from build123d import *

# Parameters (mm, degrees)
SKETCH_1_W          = 70
SKETCH_1_H          = 12
SKETCH_1_R          = 40
SKETCH_1_R_2        = 35
SKETCH_1_W_2        = 35
EXTRUDE_1_DEPTH     = 12
FILLET_1_R          = 10
SKETCH_2_R          = 2
CUT_EXTRUDE_1_DEPTH = 27
CUT_EXTRUDE_START   = -6
SKETCH_2_3_R        = 4
SKETCH_2_3_R_2      = 2
CUT_EXTRUDE_2_DEPTH = 18
EXTRUDE_START       = -12
EXTRUDE_2_DEPTH     = 12
CUT_EXTRUDE_START_2 = -12
CUT_EXTRUDE_3_DEPTH = 12
SKETCH_4_R          = 2
CUT_EXTRUDE_4_DEPTH = 67.19801074


with BuildPart() as part:
    # 스케치1 → 보스-돌출1 (new body)
    # profile 1 of 7: a face of its own
    with BuildSketch(Plane(origin=(0, 0, 0), x_dir=(0, 0, -1), z_dir=(1, 0, 0))):
        with Locations((0, -46)):
            Rectangle(SKETCH_1_W, SKETCH_1_H)
    # profile 2 of 7: a face of its own
    with BuildSketch(Plane(origin=(0, 0, 0), x_dir=(0, 0, -1), z_dir=(1, 0, 0))):
        Circle(SKETCH_1_R)
        Circle(SKETCH_1_R_2, mode=Mode.SUBTRACT)
    # profile 3 of 7: a face of its own
    with BuildSketch(Plane(origin=(0, 0, 0), x_dir=(0, 0, -1), z_dir=(1, 0, 0))):
        with BuildLine():
            ThreePointArc((-18.119935206, -35.660453561), (-26.285525679, -38.897757113), (-35, -40))
            Line((-35, -40), (0, -40))
            ThreePointArc((0, -40), (-9.316164919, -38.899988062), (-18.119935206, -35.660453561))
        make_face()
    # profile 4 of 7: a face of its own
    with BuildSketch(Plane(origin=(0, 0, 0), x_dir=(0, 0, -1), z_dir=(1, 0, 0))):
        with Locations((17.5, -46)):
            Rectangle(SKETCH_1_W_2, SKETCH_1_H)
    # profile 5 of 7: a face of its own
    with BuildSketch(Plane(origin=(0, 0, 0), x_dir=(0, 0, -1), z_dir=(1, 0, 0))):
        with BuildLine():
            ThreePointArc((18.119935206, -35.660453561), (9.316164919, -38.899988062), (0, -40))
            Line((0, -40), (35, -40))
            ThreePointArc((35, -40), (26.285525679, -38.897757113), (18.119935206, -35.660453561))
        make_face()
    # profile 6 of 7: a face of its own
    with BuildSketch(Plane(origin=(0, 0, 0), x_dir=(0, 0, -1), z_dir=(1, 0, 0))):
        with BuildLine():
            ThreePointArc((-18.119935206, -35.660453561), (-9.316164919, -38.899988062), (0, -40))
            Line((0, -40), (0, -35))
            ThreePointArc((0, -35), (-35, 0), (0, 35))
            Line((0, 35), (0, 40))
            ThreePointArc((0, 40), (-38.899988062, 9.316164919), (-18.119935206, -35.660453561))
        make_face()
    # profile 7 of 7: a face of its own
    with BuildSketch(Plane(origin=(0, 0, 0), x_dir=(0, 0, -1), z_dir=(1, 0, 0))):
        with BuildLine():
            Line((0, -35), (0, -40))
            ThreePointArc((0, -40), (9.316164919, -38.899988062), (18.119935206, -35.660453561))
            ThreePointArc((18.119935206, -35.660453561), (34.093968735, -20.918921958), (40, 0))
            ThreePointArc((40, 0), (28.284271247, 28.284271247), (0, 40))
            Line((0, 40), (0, 35))
            ThreePointArc((0, 35), (24.748737342, 24.748737342), (35, 0))
            ThreePointArc((35, 0), (24.748737342, -24.748737342), (0, -35))
        make_face()
    extrude(amount=EXTRUDE_1_DEPTH)

    # 필렛1
    # the kernel refuses this fillet: 10 mm, written as the material it adds along each edge
    with BuildSketch(Plane(origin=(0, -35.660453561, -18.119935206), x_dir=(0, -0.24898498059862248, -0.9685073460931021), z_dir=(1, 0, 0))) as fillet_1_piece_1:
        with BuildLine():
            CenterArc((19.307998012, 9.821872198), FILLET_1_R, 156.16657794, 103.002878163)
            Line((10.16075687, 13.862661663), (9.977812048, 13.943477452))
            ThreePointArc((9.977812048, 13.943477452), (5.672446884, 6.497369179), (-0.132141038, 0.150129098))
            Line((-0.132141038, 0.150129098), (-0.049796996, -0.193701469))
            ThreePointArc((-0.049796996, -0.193701469), (8.714474321, -1.302242887), (17.391367655, -0.196437444))
            Line((17.391367655, -0.196437444), (17.428948642, 0))
        make_face()
    extrude(amount=12)
    with BuildSketch(Plane(origin=(0, -35.660453561, 18.119935206), x_dir=(0, 0.6339570106071373, 0.7733682878823399), z_dir=(1, 0, 0))) as fillet_1_piece_2:
        with BuildLine():
            CenterArc((19.336075357, 9.766480968), FILLET_1_R, 154.590671351, 103.002878163)
            Line((10.303420921, 14.057303016), (10.122767833, 14.143119457))
            ThreePointArc((10.122767833, 14.143119457), (4.101387619, 7.798494651), (-0.185668093, 0.074346212))
            Line((-0.185668093, 0.074346212), (0.042969056, -0.195329619))
            ThreePointArc((0.042969056, -0.195329619), (8.59381127, 0.734076129), (17.144653483, -0.195329619))
            Line((17.144653483, -0.195329619), (17.187622539, 0))
        make_face()
    extrude(amount=12)

    # 스케치2 → 컷-돌출1 (cut)
    with BuildSketch(Plane.XZ.offset(52)):
        with Locations(Location((6, 0, 0), (0, 0, 270))):
            Circle(SKETCH_2_R)
    extrude(amount=-CUT_EXTRUDE_1_DEPTH, mode=Mode.SUBTRACT)

    # 스케치2<3> → 컷-돌출2 (cut)
    with BuildSketch(Plane.XZ.offset(52).offset(CUT_EXTRUDE_START)):
        with Locations(Location((6, 0, 0), (0, 0, 270))):
            Circle(SKETCH_2_3_R)
        with Locations(Location((6, 0, 0), (0, 0, 270))):
            Circle(SKETCH_2_3_R_2, mode=Mode.SUBTRACT)
    extrude(amount=-CUT_EXTRUDE_2_DEPTH, mode=Mode.SUBTRACT)

    # 스케치3 → 보스-돌출2 (add)
    with BuildSketch(Plane(origin=(12, 0, 0), x_dir=(0, 0, -1), z_dir=(1, 0, 0)).offset(EXTRUDE_START)):
        with BuildLine():
            ThreePointArc((26.083289209, 30.325929896), (27.202941017, 29.325756597), (28.284271247, 28.284271247))
            Line((28.284271247, 28.284271247), (33.234018716, 33.234018716))
            Line((33.234018716, 33.234018716), (31.112698372, 35.355339059))
            Line((31.112698372, 35.355339059), (26.083289209, 30.325929896))
        make_face()
        with BuildLine():
            Line((35.355339059, 31.112698372), (30.325929896, 26.083289209))
            ThreePointArc((30.325929896, 26.083289209), (31.28870697, 24.920208991), (32.206903595, 23.721622221))
            Line((32.206903595, 23.721622221), (37.476659403, 28.991378029))
            Line((37.476659403, 28.991378029), (35.355339059, 31.112698372))
        make_face()
    extrude(amount=EXTRUDE_2_DEPTH)

    # 스케치3<3> → 컷-돌출3 (cut)
    with BuildSketch(Plane(origin=(12, 0, 0), x_dir=(0, 0, -1), z_dir=(1, 0, 0)).offset(CUT_EXTRUDE_START_2)):
        with BuildLine():
            Line((28.284271247, 28.284271247), (24.748737342, 24.748737342))
            ThreePointArc((24.748737342, 24.748737342), (25.787593916, 23.664319132), (26.778976355, 22.536335668))
            Line((26.778976355, 22.536335668), (30.325929896, 26.083289209))
            ThreePointArc((30.325929896, 26.083289209), (29.325756597, 27.202941017), (28.284271247, 28.284271247))
        make_face()
    extrude(amount=CUT_EXTRUDE_3_DEPTH, mode=Mode.SUBTRACT)

    # 스케치4 → 컷-돌출4 (cut, through all)
    with BuildSketch(Plane(origin=(0, -4.242640687, -4.242640687), x_dir=(1, 0, 0), z_dir=(0, -0.7071067811865483, -0.7071067811865468))):
        with Locations(Location((6, -43.273719933, 0), (0, 0, 270))):
            Circle(SKETCH_4_R)
    extrude(amount=-CUT_EXTRUDE_4_DEPTH, mode=Mode.SUBTRACT)


solid = part.part
For this review, take the finished solid that the model builds, in its own axes (mm). A direction names the side the tool comes from. Give positions to 0.01 mm unless a question says otherwise; leave off trailing zeros. Loops run counter-clockwise (first coordinate to the right, second up) from the corner with the lowest first, then second, coordinate; pieces in that order, holes last. Notation, with made-up numbers: M -39,7.25 L -3,7.25 A15 cw -3,36.25 Z; hole C 31,63 d2. An arc over 180 degrees is marked long. Put each result on its own line as item: value. Start each with the question number.
(1) Machinability: for faces 1 (the cylindrical face through (2.095, -40.464, 0.867)), 2 (the flat face through (6, 29, -29)), 3 (the cylindrical face through (8, -49, 0)), 4 (the flat face through (4.583, 25.149, -33.634)), which of the approach directions +Z, -Z, +X, -X, +Y, -Y give a long, thin tool a straight path to every point of the face, cutting with its end or side? Answer none if there is none.
(2) Wall thickness on L1, parallel to X at y = -49.7, z = 0; L2, parallel to Y at x = 3.5, z = -29; L3, parallel to Y at x = 10.75, z = -0.5: over which ranges is each line inside the solid? List them lowest first.
(3) Add section B-B, the plane z = -8.5. Write out the cut boundary in (x, y).
(4) Add section A-A, the plane x = 6. Give the number of separate pieces and of enclosed holes in the cut face, then the cut area to 3 significant figures.
(5) For pin 1 (3.5 mm diameter, centred on x = 3.5, y = -45.5, fed in from +Z); pin 2 (4 mm diameter, centred on x = 10.5, z = -5.5, fed in from +Y); pin 3 (1.5 mm diameter, centred on x = 10.5, y = -35.5, fed in from +Z), all flat-tipped, find the tip position at first contact; note any pin that passes through.
(6) Add section C-C, the plane y = -14. Write out the cut boundary in (x, z).
(7) The part is to be moulded in two halves that separate along Z. For faces 5 (the cylindrical face through (5.23, 32.95, -30.86)), 6 (the cylindrical face through (5.9, -33.1, -29.5)), 7 (the cylindrical face through (5.92, -33.37, 29.56)), say which applies: +Z half, -Z half, draft (parallel to the pull), parting line (faces both ways), or undercut.
Result:
1. face 1: none
1. face 2: +X, -X
1. face 3: -Y
1. face 4: -Z, +X, -X
2. L1: x = 0 to 4, 8 to 12
2. L2: y = -52 to -19.6, 19.6 to 24.76, 29 to 33.24
2. L3: y = -52 to -35, 35 to 40
3. outline: M 0,-52 L 12,-52 L 12,-33.95 L 0,-33.95 Z; M 0,33.95 L 12,33.95 L 12,39.09 L 0,39.09 Z
4. separate pieces: 4
4. enclosed holes: 0
4. area: 2,170 mm^2
5. pin 1: stops at z = 35
5. pin 2: stops at y = 39.85
5. pin 3: stops at z = 30.78
6. outline: M 0,-37.47 L 12,-37.47 L 12,-32.08 L 0,-32.08 Z; M 0,32.08 L 12,32.08 L 12,37.47 L 0,37.47 Z
7. face 5: undercut
7. face 6: -Z half
7. face 7: +Z half
